Check sheet for the drawn part. Datum: minimum x, y, z corner. Units: mm. Coordinates: 2 decimals unless noted, no trailing zeros. Write each loop counter-clockwise with the first axis right and the second up, starting at its lowest first coordinate (ties: lowest second). Pieces come first, ordered by that corner, then holes. Notation, with made-up numbers: M 32.5,-16.5 L 58.5,-16.5 A10 cw 58.5,-5.5 Z; hole C -7,32.25 d2. An arc over 180 degrees is marked long. Answer in a Markdown table with one row per item.
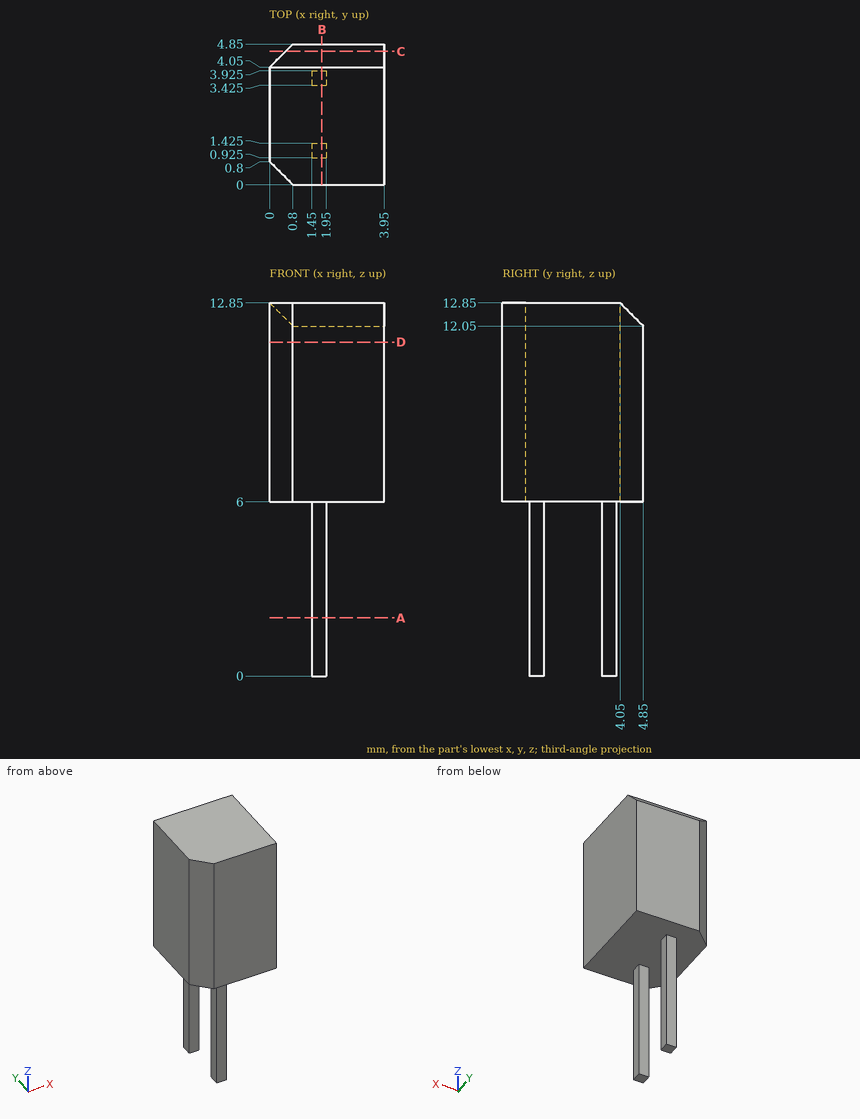
1) Thickness scan on L1, parallel to Y at x = 1.65, z = 5.75 (3 decimals); L2, parallel to Z at x = 2.15, y = 2.15; L3, parallel to X at y = 1.35, z = 2.75. Record the ranges inside material, lowest first. Write a range as [from, to].
Response values:
| item | result |
|---|---|
| L1 | y = [0.925, 1.425], [3.425, 3.925] |
| L2 | z = [6, 12.85] |
| L3 | x = [1.45, 1.95] |
2) Depth check by flat-ended pin: pin 1 (0.6 mm diameter, centred on y = 1, z = 3, fed in from -X); pin 2 (1.5 mm diameter, centred on x = 1, z = 5, fed in from -Y) (3 decimals); pin 3 (1 mm diameter, centred on x = 3, y = 3, fed in from -Z); pin 4 (1 mm diameter, centred on x = 3, z = 2, fed in from -Y). Enter the tip coordinate at first touch or a pass-through.
Response values:
| item | result |
|---|---|
| pin 1 | stops at x = 1.45 |
| pin 2 | stops at y = 0.925 |
| pin 3 | stops at z = 6 |
| pin 4 | passes through |
3) Sectioned sample at B-B (x = 1.8). Record the cut outline in (y, z) (3 decimals), then the cut area to 3 significant figures.
Response values:
| item | result |
|---|---|
| outline | M 0,6 L 0.925,6 L 0.925,0 L 1.425,0 L 1.425,6 L 3.425,6 L 3.425,0 L 3.925,0 L 3.925,6 L 4.85,6 L 4.85,12.05 L 4.05,12.85 L 0,12.85 Z |
| area | 38.9 mm² |
4) Sectioned sample at C-C (y = 4.6). Record the cut outline in (x, z).
Response values:
| item | result |
|---|---|
| outline | M 0.55,6 L 3.95,6 L 3.95,12.3 L 0.55,12.3 Z |
5) Sectioned sample at A-A (z = 2). Record the cut outline in (x, y) (3 decimals), then the cut area to 3 significant figures.
Response values:
| item | result |
|---|---|
| outline | M 1.45,0.925 L 1.95,0.925 L 1.95,1.425 L 1.45,1.425 Z; M 1.45,3.425 L 1.95,3.425 L 1.95,3.925 L 1.45,3.925 Z |
| area | 0.500 mm² |
6) Sectioned sample at D-D (z = 11.5). Record the cut outline in (x, y).
Response values:
| item | result |
|---|---|
| outline | M 0,0.8 L 0.8,0 L 3.95,0 L 3.95,4.85 L 0.8,4.85 L 0,4.05 Z |
